Source: CAD feature listing. Evaluate the final solid. Frame: model axes, mm. Face numbers are marked on the shaded views. A direction names the side the tool comes from. Round coordinates to 2 decimals unless told otherwise and drop trailing zeros. Write each loop counter-clockwise with the first axis right and the second up, starting at its lowest first coordinate (ties: lowest second). Pieces come first, ordered by that corner, then holes. Notation, with made-up numbers: (-10, 29.25) -> (36, 29.25) arc R16 ccw to (36, 50.25) -> close; hole circle Ø7 at (-33.75, 89). An arc over 180 degrees is marked (long way). Return JSON: item names as keys, results as strings. Group by question number.
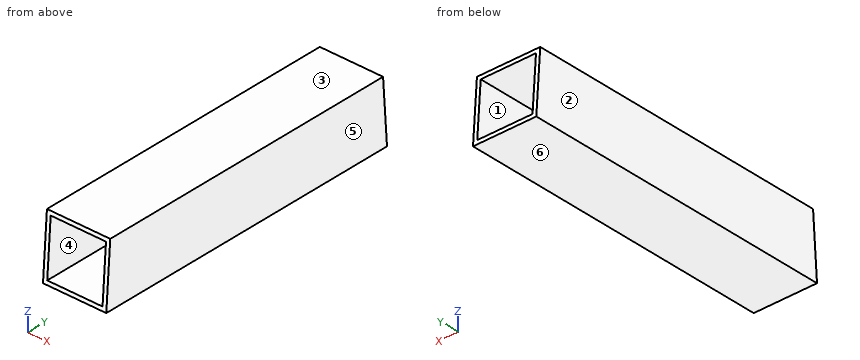
from build123d import *

# Parameters (mm, degrees)
SKETCH1_W               = 19.05
SKETCH1_H               = 19.05
BOSS_EXTRUDE1_DEPTH     = 92.1
BOSS_EXTRUDE2_DEPTH     = 19.05
CUT_EXTRUDE1_DEPTH      = 95.398144252
CUT_EXTRUDE1_DEPTH_BACK = 95.398144252
SKETCH4_W               = 16.65
SKETCH4_H               = 16.65


with BuildPart() as part:
    # Sketch1 → Boss-Extrude1 (new body)
    with BuildSketch(Plane(origin=(0, 0, 0), x_dir=(1, 0, 0), z_dir=(0, 1, 0))):
        Rectangle(SKETCH1_W, SKETCH1_H)
    extrude(amount=BOSS_EXTRUDE1_DEPTH)

    # Sketch2 → Boss-Extrude2 (add)
    with BuildSketch(Plane(origin=(9.525, 0, 0), x_dir=(0, 0, -1), z_dir=(1, 0, 0))):
        Polygon((-9.525, 92.1), (9.525, 92.1), (9.525, 93.432105768), align=None)
        Polygon((9.525, -1.332105768), (-9.525, 0), (9.525, 0), align=None)
    extrude(amount=-BOSS_EXTRUDE2_DEPTH)

    # Sketch4 → Cut-Extrude1 (cut, two sides: drawn at the far end of the back side and taken through both)
    with BuildSketch(Plane(origin=(0, 0, 0), x_dir=(1, 0, 0), z_dir=(0, 1, 0)).offset(-CUT_EXTRUDE1_DEPTH_BACK)):
        Rectangle(SKETCH4_W, SKETCH4_H)
    extrude(amount=CUT_EXTRUDE1_DEPTH + CUT_EXTRUDE1_DEPTH_BACK, mode=Mode.SUBTRACT)


solid = part.part
Item 1: Material intervals for probe 1 along X at (y, z) = (16, 8.25) (3 decimals); probe 2 along Y at (x, z) = (8.5, -2.5), sorted ascending.
Item 2: Set-up query: the marked faces 1 and 2. Return all of +Z, -Z, +X, -X, +Y, -Y with unobstructed straight access to the full face (end or side cutting, diameter ignored); none if empty.
Item 3: Pull-direction query (Z, two-part tool) for the marked faces 3, 4, 5 and 6; classes: +Z half, -Z half, draft (parallel to the pull), parting line (faces both ways), or undercut.
Item 4: Cut plane C-C on y = 53. Output: boundary loops of the cut face in (x, z) (3 decimals), and give its area (3 significant figures).
Item 5: Cut plane A-A on x = -3. Output: boundary loops of the cut face in (y, z) (3 decimals).
Item 6: Cut plane B-B on z = -0.75. Output: boundary loops of the cut face in (x, y) (1 decimal), and give its area (3 significant figures).
Here are the results:
{
 "1": {"probe 1": "x = -9.525 to -8.325, 8.325 to 9.525", "probe 2": "y = -0.84 to 92.94"},
 "2": {"face 1": "+Y, -Y", "face 2": "+Z, -Z, -X, +Y, -Y"},
 "3": {"face 3": "+Z half", "face 4": "undercut", "face 5": "draft", "face 6": "-Z half"},
 "4": {"outline": "(-9.525, -9.525) -> (9.525, -9.525) -> (9.525, 9.525) -> (-9.525, 9.525) -> close; hole (-8.325, -8.325) -> (8.325, -8.325) -> (8.325, 8.325) -> (-8.325, 8.325) -> close", "area": "85.7 mm^2"},
 "5": {"outline": "(-1.332, -9.525) -> (93.432, -9.525) -> (93.348, -8.325) -> (-1.248, -8.325) -> close; (-0.084, 8.325) -> (92.184, 8.325) -> (92.1, 9.525) -> (0, 9.525) -> close"},
 "6": {"outline": "(-9.5, -0.7) -> (-8.3, -0.7) -> (-8.3, 92.8) -> (-9.5, 92.8) -> close; (8.3, -0.7) -> (9.5, -0.7) -> (9.5, 92.8) -> (8.3, 92.8) -> close", "area": "224 mm^2"}
}
